from build123d import *

# Parameters (mm, degrees)
SKETCH_1_W      = 7
SKETCH_1_H      = 5
SKETCH_1_R      = 1.1
EXTRUDE_1_DEPTH = 5
FILLET_2_R      = 1
FILLET_1_R      = 0.25


with BuildPart() as part:
    # 草图1 → 凸台-拉伸1 (new body)
    with BuildSketch(Plane(origin=(0, 0, 0), x_dir=(1, 0, 0), z_dir=(0, 1, 0))):
        Rectangle(SKETCH_1_W, SKETCH_1_H)
        with Locations(Location((0, 0, 0), (0, 0, 270))):
            Circle(SKETCH_1_R, mode=Mode.SUBTRACT)
    extrude(amount=EXTRUDE_1_DEPTH)

    # 圆角2
    fillet_2_edges = [part.edges().sort_by_distance(p)[0] for p in [
        (3.5, 2.5, 2.5),
        (-3.5, 2.5, 2.5),
        (-3.5, 2.5, -2.5),
        (3.5, 2.5, -2.5),
    ]]
    fillet(fillet_2_edges, radius=FILLET_2_R)

    # 圆角1
    fillet_1_edges = [part.edges().sort_by_distance(p)[0] for p in [
        (0, 0, -2.5),
        (0, 5, -2.5),
        (3.5, 0, 0),
        (0, 0, 2.5),
        (-3.5, 0, 0),
        (-3.207106781, 0, -2.207106781),
        (-3.207106781, 0, 2.207106781),
        (3.207106781, 0, 2.207106781),
        (3.207106781, 0, -2.207106781),
        (3.5, 5, 0),
        (-3.5, 5, 0),
        (0, 5, 2.5),
        (-3.207106781, 5, -2.207106781),
        (-3.207106781, 5, 2.207106781),
        (3.207106781, 5, 2.207106781),
        (3.207106781, 5, -2.207106781),
    ]]
    fillet(fillet_1_edges, radius=FILLET_1_R)


solid = part.part
Source: CAD feature listing. Evaluate the final solid. Frame: model axes, mm. Round coordinates to 2 decimals unless told otherwise and drop trailing zeros. Write each loop counter-clockwise with the first axis right and the second up, starting at its lowest first coordinate (ties: lowest second). Pieces come first, ordered by that corner, then holes. Notation, with made-up numbers: (86, 24.5) - (128, 24.5) arc R27 ccw to (128, 43.5) - close; hole circle Ø11 at (88.5, 29). An arc over 180 degrees is marked (long way). Use CSV: the item, a comma, the result in double quotes. Start each with the question number.
(1) Cut plane B-B, the plane z = 0.55. Return loops of the section in (x, y).
(2) Cut plane C-C, the plane y = 4.5. Return loops of the section in (x, z).
(3) Material intervals for probe 1 along X at (y, z) = (0.8, -0.05); probe 2 along X at (y, z) = (3.3, -0.65); probe 3 along Z at (x, y) = (-0.5, 3.55), sorted ascending. Write a range as [from, to].
(4) Cut plane A-A, the plane x = 0. Return loops of the section in (y, z).
(5) Mould query, pull axis Z, two halves, no side actions, for faces 1 (the face through (0, 2, 2.5)), 2 (the face through (-3.215, 2.532, -2.199)), 3 (the face through (1.09, 2.46, -0.14)), 4 (the face through (-1, 5, -1)). Classes: pulls with the +Z half, pulls with the -Z half, needs draft (parallel to the pull), parting line crosses it, or undercut.
(6) First-contact query: pin 1 Ø1.3 at (x, z) = (0, 0) entering from -Y. Flat tip, straight axial feed; report the tip coordinate or a pass-through.
Geometry says:
1,outline,"(-3.5, 0.25) arc R0.25 ccw to (-3.25, 0) - (-0.95, 0) - (-0.95, 5) - (-3.25, 5) arc R0.25 ccw to (-3.5, 4.75) - close; (0.95, 0) - (3.25, 0) arc R0.25 ccw to (3.5, 0.25) - (3.5, 4.75) arc R0.25 ccw to (3.25, 5) - (0.95, 5) - close"
2,outline,"(-3.5, -1.5) arc R1 ccw to (-2.5, -2.5) - (2.5, -2.5) arc R1 ccw to (3.5, -1.5) - (3.5, 1.5) arc R1 ccw to (2.5, 2.5) - (-2.5, 2.5) arc R1 ccw to (-3.5, 1.5) - close; hole circle Ø2.2 at (0, 0)"
3,probe 1,"[-3.5, -1.1], [1.1, 3.5]"
3,probe 2,"[-3.5, -0.89], [0.89, 3.5]"
3,probe 3,"[-2.5, -0.98], [0.98, 2.5]"
4,outline,"(0, -2.25) arc R0.25 ccw to (0.25, -2.5) - (4.75, -2.5) arc R0.25 ccw to (5, -2.25) - (5, -1.1) - (0, -1.1) - close; (0, 1.1) - (5, 1.1) - (5, 2.25) arc R0.25 ccw to (4.75, 2.5) - (0.25, 2.5) arc R0.25 ccw to (0, 2.25) - close"
5,face 1,"pulls with the +Z half"
5,face 2,"pulls with the -Z half"
5,face 3,"undercut"
5,face 4,"needs draft"
6,pin 1,"through"
